```python
from build123d import *

# Parameters (mm, degrees)
SKETCH_1_W                       = 48
SKETCH_1_H                       = 50
SM_BASE_FLANGE_1_DEPTH           = 3
SM_EDGE_FLANGE_1_STRIP_W         = 13.4732
SM_EDGE_FLANGE_1_STRIP_H         = 3
SM_EDGE_FLANGE_1_STRIP_CUT_DEPTH = 50
SM_EDGE_FLANGE_1_DEPTH           = 50
SM_EDGE_FLANGE_2_STRIP_W         = 13.4732
SM_EDGE_FLANGE_2_STRIP_H         = 3
SM_EDGE_FLANGE_2_STRIP_CUT_DEPTH = 50
SM_EDGE_FLANGE_2_DEPTH           = 50
CHAMFER_1_SIZE                   = 5
HOLE_WIZARD_7_0_7_1_D            = 7
CUT_EXTRUDE_1_DEPTH              = 10


# Sheet-metal steps are written as plain solids
with BuildPart() as part:
    # Sketch 1 → 基体-法兰1 (new body)
    with BuildSketch(Plane.XY):
        Rectangle(SKETCH_1_W, SKETCH_1_H)
    extrude(amount=-SM_BASE_FLANGE_1_DEPTH)

    # 边线-法兰1 strip (across the edge) → 边线-法兰1 strip cut (cut)
    with BuildSketch(Plane(origin=(-24, 25, 0), x_dir=(1, 0, 0), z_dir=(0, -1, 0))):
        with Locations((-3, -1.5)):
            Rectangle(SM_EDGE_FLANGE_1_STRIP_W, SM_EDGE_FLANGE_1_STRIP_H)
    extrude(amount=SM_EDGE_FLANGE_1_STRIP_CUT_DEPTH, mode=Mode.SUBTRACT)

    # 边线-法兰1 section (across the edge) → 边线-法兰1 (add)
    with BuildSketch(Plane(origin=(-24, 25, 0), x_dir=(1, 0, 0), z_dir=(0, -1, 0))):
        with BuildLine():
            Line((0, 0.7366), (0, 21))
            Line((0, 21), (3, 21))
            Line((3, 21), (3, 0.7366))
            ThreePointArc((3, 0.7366), (3.215745145, 0.215745145), (3.7366, 0))
            Line((3.7366, 0), (3.7366, -3))
            ThreePointArc((3.7366, -3), (1.094424801, -1.905575199), (0, 0.7366))
        make_face()
    extrude(amount=SM_EDGE_FLANGE_1_DEPTH)

    # 边线-法兰2 strip (across the edge) → 边线-法兰2 strip cut (cut)
    with BuildSketch(Plane(origin=(-24, -25, 21), x_dir=(0, 0, -1), z_dir=(0, 1, 0))):
        with Locations((-3, -1.5)):
            Rectangle(SM_EDGE_FLANGE_2_STRIP_W, SM_EDGE_FLANGE_2_STRIP_H)
    extrude(amount=SM_EDGE_FLANGE_2_STRIP_CUT_DEPTH, mode=Mode.SUBTRACT)

    # 边线-法兰2 section (across the edge) → 边线-法兰2 (add)
    with BuildSketch(Plane(origin=(-24, -25, 21), x_dir=(0, 0, -1), z_dir=(0, 1, 0))):
        with BuildLine():
            Line((0, 0.7366), (0, 22))
            Line((0, 22), (3, 22))
            Line((3, 22), (3, 0.7366))
            ThreePointArc((3, 0.7366), (3.215745145, 0.215745145), (3.7366, 0))
            Line((3.7366, 0), (3.7366, -3))
            ThreePointArc((3.7366, -3), (1.094424801, -1.905575199), (0, 0.7366))
        make_face()
    extrude(amount=SM_EDGE_FLANGE_2_DEPTH)

    # 倒角1
    chamfer_1_edges = [part.edges().sort_by_distance(p)[0] for p in [
        (-46, -25, 19.5),
        (-46, 25, 19.5),
        (24, 25, -1.5),
        (24, -25, -1.5),
    ]]
    chamfer(chamfer_1_edges, length=CHAMFER_1_SIZE)

    # Ø7.0 (7) 直径孔1 (through all)
    with Locations(Plane(origin=(0, 0, -3), x_dir=(-1, 0, 0), z_dir=(0, 0, -1))):
        with Locations((-6.5, 16), (-6.5, -16)):
            Hole(HOLE_WIZARD_7_0_7_1_D / 2)

    # 草图14 → 切除-拉伸1 (cut)
    with BuildSketch(Plane(origin=(0, 0, -3), x_dir=(-1, 0, 0), z_dir=(0, 0, -1))):
        with BuildLine():
            Line((-9, 19.5), (-4, 19.5))
            ThreePointArc((-4, 19.5), (-0.5, 16), (-4, 12.5))
            Line((-4, 12.5), (-9, 12.5))
            ThreePointArc((-9, 12.5), (-12.5, 16), (-9, 19.5))
        make_face()
        with BuildLine():
            Line((-9, -12.5), (-4, -12.5))
            ThreePointArc((-4, -12.5), (-0.5, -16), (-4, -19.5))
            Line((-4, -19.5), (-9, -19.5))
            ThreePointArc((-9, -19.5), (-12.5, -16), (-9, -12.5))
        make_face()
    extrude(amount=-CUT_EXTRUDE_1_DEPTH, mode=Mode.SUBTRACT)


solid = part.part
```
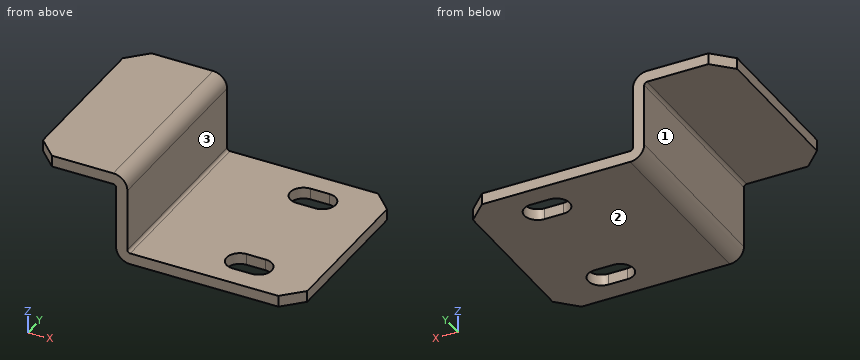
Design review of the part built by this model. Coordinates are the model's own, in mm. Face numbers are marked on the shaded views. A direction names the side the tool comes from. Coordinates: 2 decimals unless noted, no trailing zeros. Loops run counter-clockwise (first coordinate to the right, second up) from the corner with the lowest first, then second, coordinate; pieces in that order, holes last. Notation, with made-up numbers: (-27, -19.75) -> (28, -19.75) arc R18 cw to (28, -5.75) -> close; hole circle Ø5 at (-39, 7). An arc over 180 degrees is marked (long way). Answer as a JSON object with one key per item and string values.
Q1. Take a section at C-C on y = -7.5. Give the boundary of the cut face in (x, z), plus the area to 3 significant figures.
Answer block:
{"outline": "(-46, 18) -> (-24.74, 18) arc R0.74 cw to (-24, 17.26) -> (-24, 0.74) arc R3.74 ccw to (-20.26, -3) -> (24, -3) -> (24, 0) -> (-20.26, 0) arc R0.74 cw to (-21, 0.74) -> (-21, 17.26) arc R3.74 ccw to (-24.74, 21) -> (-46, 21) -> close", "area": "267 mm^2"}
Q2. Take a section at D-D on z = -1. Give the boundary of the cut face in (x, y).
Answer block:
{"outline": "(-23.57, -25) -> (19, -25) -> (24, -20) -> (24, 20) -> (19, 25) -> (-23.57, 25) -> close; hole (4, -19.5) -> (9, -19.5) arc R3.5 ccw to (9, -12.5) -> (4, -12.5) arc R3.5 ccw to start; hole (4, 12.5) -> (9, 12.5) arc R3.5 ccw to (9, 19.5) -> (4, 19.5) arc R3.5 ccw to start"}
Q3. Tool access review of the marked faces 1, 2 and 3: name each direction out of +Z, -Z, +X, -X, +Y, -Y from which nothing blocks a thin tool from reaching the whole face with its end or side.
Answer block:
{"face 1": "-Z, -X, +Y, -Y", "face 2": "-Z, +X, -X, +Y, -Y", "face 3": "+Z, +X, +Y, -Y"}
Q4. To check wall thickness, follow L1, parallel to Z at x = -11.5, y = 6; L2, parallel to X at y = 4, z = 0.75; L3, parallel to Z at x = -28.5, y = -16. State the ranges of each line that lie inside material, in increasing order.
Answer block:
{"L1": "z = -3 to 0", "L2": "x = -24 to -21", "L3": "z = 18 to 21"}
Q5. Clearance check with flat-ended pins moving along their axes: pin 1 Ø13 at (y, z) = (-9.5, 10.5) entering from -X; pin 2 Ø1 at (y, z) = (2, 6.5) entering from +X; pin 3 Ø3 at (x, y) = (-30, 0) entering from -Z. State where each tip first meets the part, or that it passes through.
Answer block:
{"pin 1": "stops at x = -24", "pin 2": "stops at x = -21", "pin 3": "stops at z = 18"}
Q6. Take a section at A-A on x = 5. Give the boundary of the cut face in (y, z), plus the area to 3 significant figures.
Answer block:
{"outline": "(-25, -3) -> (-19.5, -3) -> (-19.5, 0) -> (-25, 0) -> close; (-12.5, -3) -> (12.5, -3) -> (12.5, 0) -> (-12.5, 0) -> close; (19.5, -3) -> (25, -3) -> (25, 0) -> (19.5, 0) -> close", "area": "108 mm^2"}
Q7. Take a section at B-B on y = 16. Give the boundary of the cut face in (x, z), plus the area to 3 significant figures.
Answer block:
{"outline": "(-46, 18) -> (-24.74, 18) arc R0.74 cw to (-24, 17.26) -> (-24, 0.74) arc R3.74 ccw to (-20.26, -3) -> (0.5, -3) -> (0.5, 0) -> (-20.26, 0) arc R0.74 cw to (-21, 0.74) -> (-21, 17.26) arc R3.74 ccw to (-24.74, 21) -> (-46, 21) -> close; (12.5, -3) -> (24, -3) -> (24, 0) -> (12.5, 0) -> close", "area": "231 mm^2"}
